Design review of the part built by this model. Coordinates are the model's own, in mm. Coordinates: 2 decimals unless noted, no trailing zeros. Loops run counter-clockwise (first coordinate to the right, second up) from the corner with the lowest first, then second, coordinate; pieces in that order, holes last.
Q1. For P1, Ø8, axis at x = 15, z = -29, coming from the -Y side; P2, Ø9, axis at x = 26.16, z = 19.95, coming from the +Y side, all flat-tipped, find the tip position at first contact; note any pin that passes through.
Q2. Add section C-C on z = 0. Give the boundary of the cut face in (x, y) (3 decimals).
Q3. Wall thickness on probe 1 along X at (y, z) = (9.05, -19.95) (3 decimals); probe 2 along X at (y, z) = (4, -19.95) (3 decimals); probe 3 along Z at (x, y) = (-26.16, 4.25): over which ranges is each line inside the solid? List them lowest first.
Q4. Add section D-D on x = 26.16. Give the boundary of the cut face in (y, z) (3 decimals).
Q5. Add section A-A on x = 0. Give the boundary of the cut face in (y, z) (3 decimals).
Q6. Add section B-B on y = 1.5. Give the boundary of the cut face in (x, z) (3 decimals).
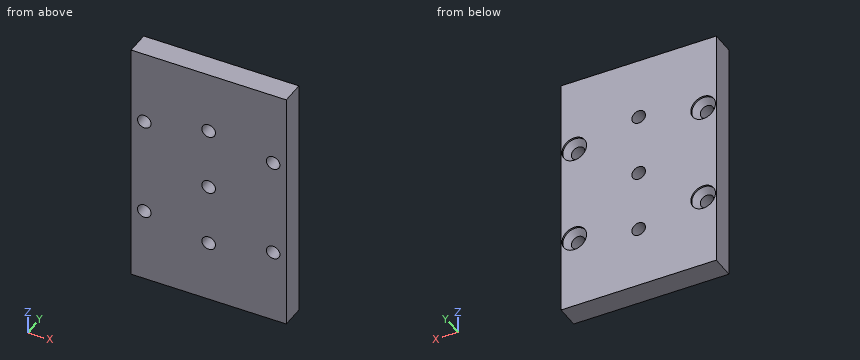
```python
from build123d import *

# Parameters (mm, degrees)
ESBO_O1_W                       = 63.01
ESBO_O1_H                       = 100
RESSALTO_EXTRUS_O1_DEPTH        = 9.525
ESBO_O2_R                       = 2.75
CORTE_EXTRUS_O1_DEPTH           = 10
ESBO_O3_R                       = 5
CORTE_EXTRUS_O2_DEPTH           = 0.7
ESBO_O4_R                       = 5
CORTE_EXTRUS_O3_DEPTH           = 2.5
CORTE_EXTRUS_O3_DRAFT           = -45
CORTE_EXTRUS_O3_PROFILE_2_DEPTH = 2.5
CORTE_EXTRUS_O3_PROFILE_2_DRAFT = -45
CORTE_EXTRUS_O3_PROFILE_3_DEPTH = 2.5
CORTE_EXTRUS_O3_PROFILE_3_DRAFT = -45
CORTE_EXTRUS_O3_PROFILE_4_DEPTH = 2.5
CORTE_EXTRUS_O3_PROFILE_4_DRAFT = -45


with BuildPart() as part:
    # Esboço1 → Ressalto-extrusão1 (new body)
    with BuildSketch(Plane(origin=(0, 0, 0), x_dir=(1, 0, 0), z_dir=(0, 1, 0))):
        Rectangle(ESBO_O1_W, ESBO_O1_H)
    extrude(amount=RESSALTO_EXTRUS_O1_DEPTH)

    # Esboço2 → Corte-extrusão1 (cut)
    with BuildSketch(Plane.XZ):
        with Locations(Location((-26.16, 19.950903247, 0), (0, 0, 270))):
            Circle(ESBO_O2_R)
        with Locations(Location((0, 25, 0), (0, 0, 270))):
            Circle(ESBO_O2_R)
        with Locations(Location((26.16, 19.950903247, 0), (0, 0, 270))):
            Circle(ESBO_O2_R)
        with Locations(Location((0, 0, 0), (0, 0, 270))):
            Circle(ESBO_O2_R)
        with Locations(Location((-26.16, -19.95, 0), (0, 0, 270))):
            Circle(ESBO_O2_R)
        with Locations(Location((0, -25, 0), (0, 0, 270))):
            Circle(ESBO_O2_R)
        with Locations(Location((26.16, -19.95, 0), (0, 0, 270))):
            Circle(ESBO_O2_R)
    extrude(amount=-CORTE_EXTRUS_O1_DEPTH, mode=Mode.SUBTRACT)

    # Esboço3 → Corte-extrusão2 (cut)
    with BuildSketch(Plane(origin=(0, 9.525, 0), x_dir=(1, 0, 0), z_dir=(0, 1, 0))):
        with Locations(Location((26.16, 19.95, 0), (0, 0, 270))):
            Circle(ESBO_O3_R)
        with Locations(Location((26.16, -19.950903247, 0), (0, 0, 270))):
            Circle(ESBO_O3_R)
        with Locations(Location((-26.16, -19.950903247, 0), (0, 0, 270))):
            Circle(ESBO_O3_R)
        with Locations(Location((-26.16, 19.95, 0), (0, 0, 270))):
            Circle(ESBO_O3_R)
    extrude(amount=-CORTE_EXTRUS_O2_DEPTH, mode=Mode.SUBTRACT)


with BuildPart() as corte_extrus_o3_tool:
    # Esboço4 → Corte-extrusão3 (with draft: the straight prism first)
    with BuildSketch(Plane(origin=(0, 8.825, 0), x_dir=(1, 0, 0), z_dir=(0, 1, 0))):
        with Locations(Location((26.16, 19.95, 0), (0, 0, 270))):
            Circle(ESBO_O4_R)
    extrude(amount=-CORTE_EXTRUS_O3_DEPTH)
    # Corte-extrusão3: the draft: its side faces are tilted about the plane it starts from
    corte_extrus_o3_sides = [corte_extrus_o3_tool.faces().sort_by_distance(p)[0] for p in [
        (26.16, 7.575, -24.95),
    ]]
    draft(corte_extrus_o3_sides, Plane(origin=(0, 8.825, 0), x_dir=(1, 0, 0), z_dir=(0, 1, 0)), CORTE_EXTRUS_O3_DRAFT)


with BuildPart() as part_1:
    add(part.part)

    # Corte-extrusão3: cut by corte_extrus_o3_tool
    add(corte_extrus_o3_tool.part, mode=Mode.SUBTRACT)


with BuildPart() as corte_extrus_o3_profile_2_tool:
    # Esboço4 → Corte-extrusão3 profile 2 (with draft: the straight prism first)
    with BuildSketch(Plane(origin=(0, 8.825, 0), x_dir=(1, 0, 0), z_dir=(0, 1, 0))):
        with Locations(Location((-26.16, 19.95, 0), (0, 0, 270))):
            Circle(ESBO_O4_R)
    extrude(amount=-CORTE_EXTRUS_O3_PROFILE_2_DEPTH)
    # Corte-extrusão3 profile 2: the draft: its side faces are tilted about the plane it starts from
    corte_extrus_o3_profile_2_sides = [corte_extrus_o3_profile_2_tool.faces().sort_by_distance(p)[0] for p in [
        (-26.16, 7.575, -24.95),
    ]]
    draft(corte_extrus_o3_profile_2_sides, Plane(origin=(0, 8.825, 0), x_dir=(1, 0, 0), z_dir=(0, 1, 0)), CORTE_EXTRUS_O3_PROFILE_2_DRAFT)


with BuildPart() as part_2:
    add(part_1.part)

    # Corte-extrusão3 profile 2: cut by corte_extrus_o3_profile_2_tool
    add(corte_extrus_o3_profile_2_tool.part, mode=Mode.SUBTRACT)


with BuildPart() as corte_extrus_o3_profile_3_tool:
    # Esboço4 → Corte-extrusão3 profile 3 (with draft: the straight prism first)
    with BuildSketch(Plane(origin=(0, 8.825, 0), x_dir=(1, 0, 0), z_dir=(0, 1, 0))):
        with Locations(Location((-26.16, -19.950903247, 0), (0, 0, 270))):
            Circle(ESBO_O4_R)
    extrude(amount=-CORTE_EXTRUS_O3_PROFILE_3_DEPTH)
    # Corte-extrusão3 profile 3: the draft: its side faces are tilted about the plane it starts from
    corte_extrus_o3_profile_3_sides = [corte_extrus_o3_profile_3_tool.faces().sort_by_distance(p)[0] for p in [
        (-26.16, 7.575, 14.950903247),
    ]]
    draft(corte_extrus_o3_profile_3_sides, Plane(origin=(0, 8.825, 0), x_dir=(1, 0, 0), z_dir=(0, 1, 0)), CORTE_EXTRUS_O3_PROFILE_3_DRAFT)


with BuildPart() as part_3:
    add(part_2.part)

    # Corte-extrusão3 profile 3: cut by corte_extrus_o3_profile_3_tool
    add(corte_extrus_o3_profile_3_tool.part, mode=Mode.SUBTRACT)


with BuildPart() as corte_extrus_o3_profile_4_tool:
    # Esboço4 → Corte-extrusão3 profile 4 (with draft: the straight prism first)
    with BuildSketch(Plane(origin=(0, 8.825, 0), x_dir=(1, 0, 0), z_dir=(0, 1, 0))):
        with Locations(Location((26.16, -19.950903247, 0), (0, 0, 270))):
            Circle(ESBO_O4_R)
    extrude(amount=-CORTE_EXTRUS_O3_PROFILE_4_DEPTH)
    # Corte-extrusão3 profile 4: the draft: its side faces are tilted about the plane it starts from
    corte_extrus_o3_profile_4_sides = [corte_extrus_o3_profile_4_tool.faces().sort_by_distance(p)[0] for p in [
        (26.16, 7.575, 14.950903247),
    ]]
    draft(corte_extrus_o3_profile_4_sides, Plane(origin=(0, 8.825, 0), x_dir=(1, 0, 0), z_dir=(0, 1, 0)), CORTE_EXTRUS_O3_PROFILE_4_DRAFT)


with BuildPart() as part_4:
    add(part_3.part)

    # Corte-extrusão3 profile 4: cut by corte_extrus_o3_profile_4_tool
    add(corte_extrus_o3_profile_4_tool.part, mode=Mode.SUBTRACT)


solid = part_4.part
```
Entries:
1. P1: stops at y = 0
1. P2: stops at y = 8.33
2. outline: (-31.505, 0) - (-2.75, 0) - (-2.75, 9.525) - (-31.505, 9.525) - close; (2.75, 0) - (31.505, 0) - (31.505, 9.525) - (2.75, 9.525) - close
3. probe 1: x = -31.505 to -31.16, -21.16 to 21.16, 31.16 to 31.505
3. probe 2: x = -31.505 to -28.91, -23.41 to 23.41, 28.91 to 31.505
3. probe 3: z = -50 to -22.7, -17.2 to 17.2, 22.7 to 50
4. outline: (0, -50) - (9.525, -50) - (9.525, -24.95) - (8.825, -24.95) - (6.575, -22.7) - (0, -22.7) - close; (0, -17.2) - (6.575, -17.2) - (8.825, -14.95) - (9.525, -14.95) - (9.525, 14.951) - (8.825, 14.951) - (6.575, 17.201) - (0, 17.201) - close; (0, 22.701) - (6.575, 22.701) - (8.825, 24.951) - (9.525, 24.951) - (9.525, 50) - (0, 50) - close
5. outline: (0, -50) - (9.525, -50) - (9.525, -27.75) - (0, -27.75) - close; (0, -22.25) - (9.525, -22.25) - (9.525, -2.75) - (0, -2.75) - close; (0, 2.75) - (9.525, 2.75) - (9.525, 22.25) - (0, 22.25) - close; (0, 27.75) - (9.525, 27.75) - (9.525, 50) - (0, 50) - close
6. outline: (-31.505, -50) - (31.505, -50) - (31.505, 50) - (-31.505, 50) - close; hole circle Ø5.5 at (-26.16, -19.95); hole circle Ø5.5 at (-26.16, 19.951); hole circle Ø5.5 at (0, -25); hole circle Ø5.5 at (0, 0); hole circle Ø5.5 at (0, 25); hole circle Ø5.5 at (26.16, -19.95); hole circle Ø5.5 at (26.16, 19.951)
